from build123d import *

# Parameters (mm, degrees)
SALIENTE_EXTRUIR1_DEPTH      = 3
CROQUIS2_R                   = 1.5
CORTAR_EXTRUIR1_DEPTH        = 3
CROQUIS3_R                   = 1.5
CORTAR_EXTRUIR2_DEPTH        = 3
SALIENTE_EXTRUIR2_DEPTH      = 18
SALIENTE_EXTRUIR2_DEPTH_BACK = 3
CROQUIS5_R                   = 1.5
CORTAR_EXTRUIR3_DEPTH        = 3
CROQUIS6_R                   = 1.5
CORTAR_EXTRUIR4_DEPTH        = 3


with BuildPart() as part:
    # Croquis1 → Saliente-Extruir1 (new body)
    with BuildSketch(Plane(origin=(0, 0, 0), x_dir=(1, 0, 0), z_dir=(0, 1, 0))):
        Polygon((0, 0), (62, 0), (123.449927666, 46.399422301), (128.270646866, 40.015014231), (64.681080335, -8), (0, -8), align=None)
    extrude(amount=SALIENTE_EXTRUIR1_DEPTH)

    # Croquis2 → Cortar-Extruir1 (cut)
    with BuildSketch(Plane(origin=(0, 3, 0), x_dir=(1, 0, 0), z_dir=(0, 1, 0))):
        with Locations(Location((8, -4, 0), (0, 0, 270))):
            Circle(CROQUIS2_R)
        with Locations(Location((54, -4, 0), (0, 0, 270))):
            Circle(CROQUIS2_R)
    extrude(amount=-CORTAR_EXTRUIR1_DEPTH, mode=Mode.SUBTRACT)

    # Croquis3 → Cortar-Extruir2 (cut)
    with BuildSketch(Plane(origin=(0, 3, 0), x_dir=(1, 0, 0), z_dir=(0, 1, 0))):
        with Locations(Location((70.794767669, 1.628515165, 0), (0, 0, 270))):
            Circle(CROQUIS3_R)
        with Locations(Location((119.475879197, 38.386499066, 0), (0, 0, 270))):
            Circle(CROQUIS3_R)
    extrude(amount=-CORTAR_EXTRUIR2_DEPTH, mode=Mode.SUBTRACT)

    # Croquis4 → Saliente-Extruir2 (add, two sides: drawn at the far end of the back side and taken through both)
    with BuildSketch(Plane(origin=(0, 3, 0), x_dir=(1, 0, 0), z_dir=(0, 1, 0)).offset(-SALIENTE_EXTRUIR2_DEPTH_BACK)):
        Polygon((0, 0), (0, 3), (60.994594874, 3), (121.642157966, 48.793575327), (123.449927666, 46.399422301), (62, 0), align=None)
    extrude(amount=SALIENTE_EXTRUIR2_DEPTH + SALIENTE_EXTRUIR2_DEPTH_BACK)

    # Croquis5 → Cortar-Extruir3 (cut)
    with BuildSketch(Plane.XY):
        with Locations((8, 13.5)):
            Circle(CROQUIS5_R)
        with Locations((54, 13.5)):
            Circle(CROQUIS5_R)
    extrude(amount=-CORTAR_EXTRUIR3_DEPTH, mode=Mode.SUBTRACT)

    # Croquis6 → Cortar-Extruir4 (cut)
    with BuildSketch(Plane(origin=(22.513104431, 0, 29.815643605), x_dir=(0.798051008651339, 0, -0.6025899000071112), z_dir=(0.6025899000071112, 0, 0.798051008651339))):
        with Locations((57.479162536, 13.5)):
            Circle(CROQUIS6_R)
        with Locations((118.479162536, 13.5)):
            Circle(CROQUIS6_R)
    extrude(amount=-CORTAR_EXTRUIR4_DEPTH, mode=Mode.SUBTRACT)


solid = part.part
Input: part model. Units: mm. Frame: model coordinates. A direction names the side the tool comes from. Coordinates: 2 decimals unless noted, no trailing zeros. Write each loop counter-clockwise with the first axis right and the second up, starting at its lowest first coordinate (ties: lowest second). Pieces come first, ordered by that corner, then holes. Notation, with made-up numbers: M 79.25,52 L 115.25,52 A35 cw 115.25,88 Z; hole C -26.75,-7.5 d5. An arc over 180 degrees is marked long. Answer as a JSON object with one key per item and string values. Group by question number.
(1) Section B-B on z = 4. Output: boundary loops of the cut face in (x, y).
(2) Section D-D on y = 7. Output: boundary loops of the cut face in (x, z).
(3) Section A-A on x = 54. Output: boundary loops of the cut face in (y, z), plus the area to 3 significant figures.
(4) Ray query, line 1 along Y through (x, z) = (8, -0.9); line 2 along X through (y, z) = (2.25, 4); line 3 along Z through (x, y) = (13.5, 15). Return the intervals inside material, ascending. Write a range as [from, to].
(5) Contact query for flat-ended pins moving along their axis: P1, Ø5.5, axis at x = 20.5, y = 15, coming from the +Z side; P2, Ø3.5, axis at x = 70.79, z = -1.63, coming from the -Y side; P3, Ø12, axis at x = 95, y = 5, coming from the -Z side; P4, Ø1, axis at x = 27.5, z = 1.5, coming from the +Y side. Output: stop coordinate, or through.
(6) Set-up query: faces 4 (the face through (93.155, 11.874, -23.525)), 5 (the face through (31, 12, 0)), 6 (the face through (30, 10, -3)). Return all of +Z, -Z, +X, -X, +Y, -Y with unobstructed straight access to the full face (end or side cutting, diameter ignored); none if empty.
(7) Mould query, pull axis Y, two halves, no side actions, for faces 1 (the face through (69, 3, -5)), 2 (the face through (55.43, 13.95, -1.48)), 3 (the face through (6.67, 1.52, 4.69)). Classes: pulls with the +Y half, pulls with the -Y half, needs draft (parallel to the pull), parting line crosses it, or undercut.
(8) Section C-C on y = 13.5. Output: boundary loops of the cut face in (x, z), plus the area to 3 significant figures.
Result set:
{
 "1": {"outline": "M 0,0 L 6.5,0 L 6.5,3 L 0,3 Z; M 9.5,0 L 52.5,0 L 52.5,3 L 9.5,3 Z; M 55.5,0 L 69.98,0 L 69.98,3 L 55.5,3 Z"},
 "2": {"outline": "M 0,-3 L 60.99,-3 L 121.64,-48.79 L 123.45,-46.4 L 62,0 L 0,0 Z"},
 "3": {"outline": "M 0,-3 L 12,-3 L 12,0 L 3,0 L 3,2.5 L 0,2.5 Z; M 0,5.5 L 3,5.5 L 3,8 L 0,8 Z; M 15,-3 L 21,-3 L 21,0 L 15,0 Z", "area": "69.0 mm2"},
 "4": {"line 1": "y = [0, 12], [15, 21]", "line 2": "x = [0, 6.5], [9.5, 52.5], [55.5, 69.98]", "line 3": "z = [-3, 0]"},
 "5": {"P1": "stops at z = 0", "P2": "stops at y = 0", "P3": "stops at z = -33.21", "P4": "stops at y = 3"},
 "6": {"face 4": "+Z, +X, +Y", "face 5": "+Z, +X, -X, +Y", "face 6": "-Z, -X, +Y, -Y"},
 "7": {"face 1": "pulls with the +Y half", "face 2": "undercut", "face 3": "needs draft"},
 "8": {"outline": "M 0,-3 L 6.5,-3 L 6.5,0 L 0,0 Z; M 9.5,-3 L 52.5,-3 L 52.5,0 L 9.5,0 Z; M 55.5,-3 L 60.99,-3 L 65.38,-6.31 L 67.19,-3.92 L 62,0 L 55.5,0 Z; M 67.77,-8.12 L 114.06,-43.07 L 115.87,-40.67 L 69.58,-5.72 Z; M 116.45,-44.88 L 121.64,-48.79 L 123.45,-46.4 L 118.26,-42.48 Z", "area": "378 mm2"}
}
